The listing builds one solid part. Answer for the finished solid, in the listing's coordinates (mm). A direction names the side the tool comes from. Coordinates: 2 decimals unless noted, no trailing zeros. Loops run counter-clockwise (first coordinate to the right, second up) from the corner with the lowest first, then second, coordinate; pieces in that order, holes last. Notation, with made-up numbers: M 62,75 L 81,75 A37 ccw 81,114 Z; hole C 52.25,-30 d2. An arc over 180 degrees is marked long. Answer as a JSON object with one key per item and string values. Group by question number.
1. A cutting plane is placed at C-C on z = -7.25. Give the vertices of the cut face in (x, y).
2. Determine the mould class of faces 3 (the face through (-7.559, -5.796, 5.984)), 4 (the face through (11, 6, 0)), 5 (the face through (4.76, -0.09, 7.96)) for opening direction Y: released by +Y, released by -Y, zero draft, split by the parting line, or undercut.
3. For faces 1 (the face through (0, 0, 9.525)), 2 (the face through (3, 0, 6.35)), determine the directions among +Z, -Z, +X, -X, +Y, -Y from which every point of the face is accessible in a straight line to the end or side of a thin tool.
4. Given pin 1 (1.6 mm diameter, centred on y = 1.5, z = 8.5, fed in from +X); pin 2 (6 mm diameter, centred on x = -12.5, z = -8.5, fed in from +Y); pin 3 (1.5 mm diameter, centred on x = -5, y = 14.5, fed in from +Z), each flat-ended and moving along its own axis, determine where each tip first touches the part or whether it passes through.
5. A cutting plane is placed at B-B on x = 0. Give the vertices of the cut face in (y, z) (3 decimals), and give its area (3 significant figures).
6. A cutting plane is placed at D-D on y = 16. Give the vertices of the cut face in (x, z) (3 decimals), and give its area (3 significant figures).
7. Straight lines are drawn through the part: L1, parallel to Z at x = -1, y = -13.5 (3 decimals); L2, parallel to Y at x = 0.5, z = -3.5; L3, parallel to Y at x = 8, z = -3.25. For each, find the intervals that lie inside material, in ascending order.
from build123d import *

# Parameters (mm, degrees)
SKETCH1_R           = 25.4
BOSS_EXTRUDE1_DEPTH = 15.875
SKETCH2_R           = 9.525
BOSS_EXTRUDE2_DEPTH = 9.525
FILLET2_R           = 2.54
CUT_EXTRUDE1_DEPTH  = 3.175


with BuildPart() as part:
    # Sketch1 → Boss-Extrude1 (new body)
    with BuildSketch(Plane.XY):
        Circle(SKETCH1_R)
    extrude(amount=-BOSS_EXTRUDE1_DEPTH)

    # Sketch2 → Boss-Extrude2 (add)
    with BuildSketch(Plane.XY):
        Circle(SKETCH2_R)
    extrude(amount=BOSS_EXTRUDE2_DEPTH)

    # Fillet2
    fillet2_edges = [part.edges().sort_by_distance(p)[0] for p in [
        (-9.525, 0, 0),
    ]]
    fillet(fillet2_edges, radius=FILLET2_R)

    # Sketch3 → Cut-Extrude1 (cut)
    with BuildSketch(Plane.XY.offset(9.525)):
        with BuildLine():
            Line((-1.27, 4.590044254), (-1.27, -4.590044254))
            ThreePointArc((-1.27, -4.590044254), (-4.7625, 0), (-1.27, 4.590044254))
        make_face()
        with BuildLine():
            Line((1.27, 4.590044254), (1.27, -4.590044254))
            ThreePointArc((1.27, -4.590044254), (4.7625, 0), (1.27, 4.590044254))
        make_face()
    extrude(amount=-CUT_EXTRUDE1_DEPTH, mode=Mode.SUBTRACT)


solid = part.part
From the geometry:
{
 "1": {"outline": "C 0,0 d50.8"},
 "2": {"face 3": "split by the parting line", "face 4": "zero draft", "face 5": "undercut"},
 "3": {"face 1": "+Z, +X, -X, +Y, -Y", "face 2": "+Z"},
 "4": {"pin 1": "stops at x = 9.5", "pin 2": "stops at y = 23.56", "pin 3": "stops at z = 0"},
 "5": {"outline": "M -25.4,-15.875 L 25.4,-15.875 L 25.4,0 L 12.065,0 A2.54 cw 9.525,2.54 L 9.525,9.525 L -9.525,9.525 L -9.525,2.54 A2.54 cw -12.065,0 L -25.4,0 Z", "area": "991 mm²"},
 "6": {"outline": "M -19.727,-15.875 L 19.727,-15.875 L 19.727,0 L -19.727,0 Z", "area": "626 mm²"},
 "7": {"L1": "z = -15.875 to 0", "L2": "y = -25.4 to 25.4", "L3": "y = -24.11 to 24.11"}
}
